Autodesk Inventor part; units mm, degrees
ref_plane "YZ Plane" through (0, 0, 0) normal (1, 0, 0) x (0, 1, 0)
ref_plane "XZ Plane" through (0, 0, 0) normal (0, 1, 0) x (-1, 0, 0)
ref_plane "XY Plane" through (0, 0, 0) normal (0, 0, 1) x (1, 0, 0)
sketch "草圖1" plane through (0, 0, 0) normal (0, 0, 1) x (1, 0, 0)
  line L0 (-50, 50) -> (50, 50)
  line L1 (50, 50) -> (50, -50)
  line L2 (50, -50) -> (-50, -50)
  line L3 (-50, -50) -> (-50, 50)
  point P0 (0, 0)
  dimension "d0" = 100
  dimension "d1" = 100
  dimension "d2" = 50
  dimension "d3" = 50
extrude "擠出1" add sketch "草圖1" along normal blind 100
sketch "草圖2" plane through (0, 0, 100) normal (0, 0, 1) x (1, 0, 0)
  line L0 (-40, 40) -> (40, 40)
  line L1 (40, 40) -> (40, -40)
  line L2 (40, -40) -> (-40, -40)
  line L3 (-40, -40) -> (-40, 40)
  point P0 (0, 0)
  dimension "d6" = 80
  dimension "d7" = 80
  dimension "d8" = 40
  dimension "d9" = 40
extrude "擠出2" cut sketch "草圖2" against normal blind 90
fillet "圓角1" radius 5 4 edges at (-50, -50, 50) (50, -50, 50) (50, 50, 50) (-50, 50, 50)
fillet "圓角2" radius 1 20 edges at (-48.5355, 48.5355, 100) (-50, 0, 100) (-48.5355, -48.5355, 100) (0, -50, 100) (48.5355, -48.5355, 100) (50, 0, 100) (48.5355, 48.5355, 100) (0, 50, 100) (0, 40, 100) (40, 0, 100) (0, -40, 100) (-40, 0, 100) (-48.5355, 48.5355, 0) (0, 50, 0) (48.5355, 48.5355, 0) (50, 0, 0) (48.5355, -48.5355, 0) (0, -50, 0) (-48.5355, -48.5355, 0) (-50, 0, 0)
properties part number "遙控器盒"
Could you check a few things on this model? Use its own coordinates, in mm. A direction names the side the tool comes from. Round coordinates to 2 decimals unless told otherwise and drop trailing zeros. Loops run counter-clockwise (first coordinate to the right, second up) from the corner with the lowest first, then second, coordinate; pieces in that order, holes last.
Q1. On a 3-axis mill with a long thin cutter (end or side, diameter ignored), from which of +Z, -Z, +X, -X, +Y, -Y can I reach the whole of each face in a straight line? I mean faces 1 (the flat face through (1, -50, 49)), 2 (the flat face through (-40, -1, 55)). Say none if no direction works.
Q2. I want a section at A-A (z = 34). Write out the boundary of the cut face in (x, y).
Q3. For P1, Ø4, axis at x = -22, y = -27.5, coming from the -Z side; P2, Ø2, axis at x = 25.5, y = 16.5, coming from the +Z side, each with a flat end and sliding along its axis, tell me the tip position at first contact or that it passes through.
Q4. Please list where these lines run through material, in increasing order: L1, parallel to Y at x = 22.5, z = 65; L2, parallel to Z at x = 30, y = 38.5.
Q5. I want a section at B-B (y = -17.5). Write out the boundary of the cut face in (x, z), and give its area (3 significant figures).
Answer below:
1. face 1: +Z, -Z, +X, -X, -Y
1. face 2: +Z
2. outline: (-50, -45) arc R5 ccw to (-45, -50) - (45, -50) arc R5 ccw to (50, -45) - (50, 45) arc R5 ccw to (45, 50) - (-45, 50) arc R5 ccw to (-50, 45) - close; hole (-40, -40) - (40, -40) - (40, 40) - (-40, 40) - close
3. P1: stops at z = 0
3. P2: stops at z = 10
4. L1: y = -50 to -40, 40 to 50
4. L2: z = 0 to 10
5. outline: (-50, 1) arc R1 ccw to (-49, 0) - (49, 0) arc R1 ccw to (50, 1) - (50, 99) arc R1 ccw to (49, 100) - (41, 100) arc R1 ccw to (40, 99) - (40, 10) - (-40, 10) - (-40, 99) arc R1 ccw to (-41, 100) - (-49, 100) arc R1 ccw to (-50, 99) - close
5. area: 2,800 mm2
